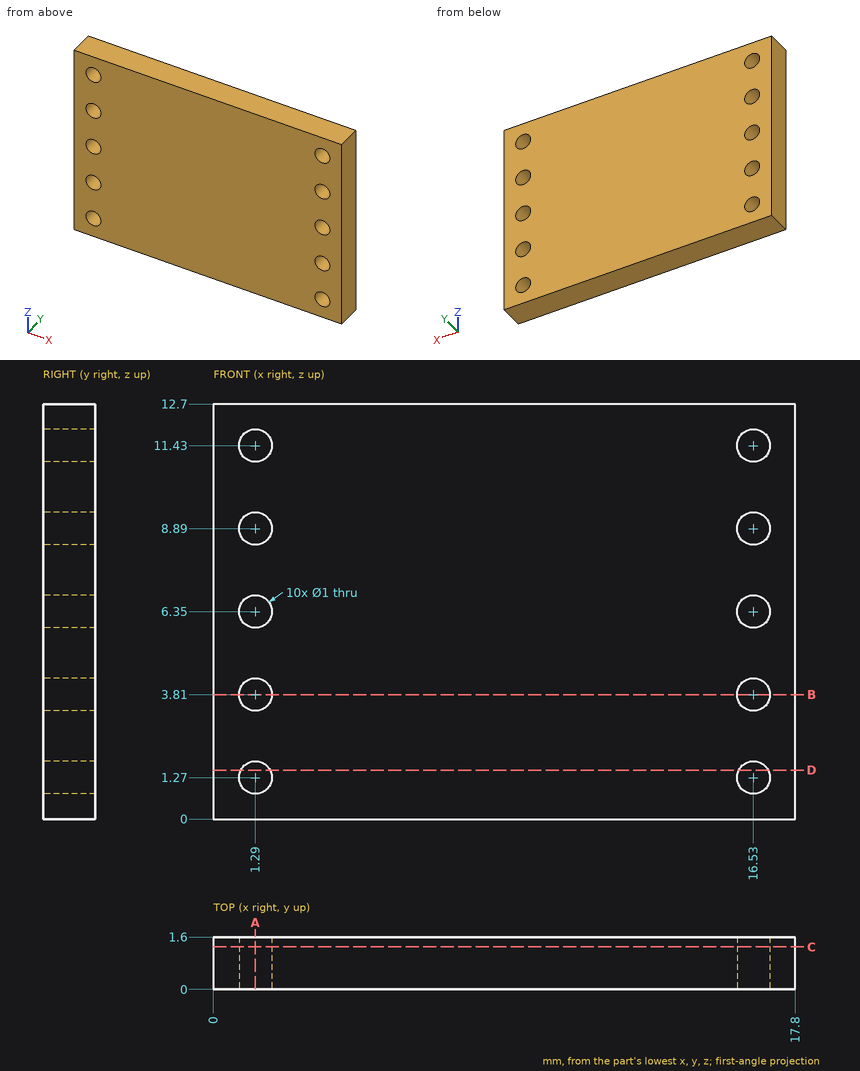
The drawing under review shows one solid part. Ordinate dimensions are in mm from its lowest x, y, z. Coordinates: 2 decimals unless noted, no trailing zeros. Order: outer loops, then holes, each group sorted by start corner. A loop starts at its lowest first (then second) coordinate and runs counter-clockwise, first axis right, second up. Notation, with made-up numbers: M 71,-39.75 L 89,-39.75 A15 cw 89,-30.75 Z; hole C -27.75,15.5 d6. An arc over 180 degrees is marked long. Use a Markdown table: item, result.
(1) Add section A-A (x = 1.29). Give the boundary of the cut face in (y, z).
Worked answers:
| item | result |
|---|---|
| outline | M 0,0 L 1.6,0 L 1.6,0.77 L 0,0.77 Z; M 0,1.77 L 1.6,1.77 L 1.6,3.31 L 0,3.31 Z; M 0,4.31 L 1.6,4.31 L 1.6,5.85 L 0,5.85 Z; M 0,6.85 L 1.6,6.85 L 1.6,8.39 L 0,8.39 Z; M 0,9.39 L 1.6,9.39 L 1.6,10.93 L 0,10.93 Z; M 0,11.93 L 1.6,11.93 L 1.6,12.7 L 0,12.7 Z |
(2) Wall thickness on probe 1 along X at (y, z) = (0.8, 1.25); probe 2 along Z at (x, y) = (1.29, 0.9); probe 3 along X at (y, z) = (0.75, 4): over which ranges is each line inside the solid? List them lowest first.
Worked answers:
| item | result |
|---|---|
| probe 1 | x = 0 to 0.79, 1.79 to 16.03, 17.03 to 17.8 |
| probe 2 | z = 0 to 0.77, 1.77 to 3.31, 4.31 to 5.85, 6.85 to 8.39, 9.39 to 10.93, 11.93 to 12.7 |
| probe 3 | x = 0 to 0.83, 1.75 to 16.07, 16.99 to 17.8 |
(3) Add section B-B (z = 3.81). Give the boundary of the cut face in (x, y), then the cut area to 3 significant figures.
Worked answers:
| item | result |
|---|---|
| outline | M 0,0 L 0.79,0 L 0.79,1.6 L 0,1.6 Z; M 1.79,0 L 16.03,0 L 16.03,1.6 L 1.79,1.6 Z; M 17.03,0 L 17.8,0 L 17.8,1.6 L 17.03,1.6 Z |
| area | 25.3 mm2 |
(4) Add section D-D (z = 1.5). Give the boundary of the cut face in (x, y).
Worked answers:
| item | result |
|---|---|
| outline | M 0,0 L 0.85,0 L 0.85,1.6 L 0,1.6 Z; M 1.73,0 L 16.09,0 L 16.09,1.6 L 1.73,1.6 Z; M 16.97,0 L 17.8,0 L 17.8,1.6 L 16.97,1.6 Z |
(5) Add section C-C (y = 1.3). Count the separate pieces of the cut face and the enclosed holes in it, then the cut area to 3 significant figures.
Worked answers:
| item | result |
|---|---|
| separate pieces | 1 |
| enclosed holes | 10 |
| area | 218 mm2 |
